Source: three-view drawing plus pictorial views. Frame: mm from the lowest corner of the part. A direction names the side the tool comes from. Give positions to 0.01 mm unless a question says otherwise; leave off trailing zeros. Loops run counter-clockwise (first coordinate to the right, second up) from the corner with the lowest first, then second, coordinate; pieces in that order, holes last.
1. Material intervals for line 1 along X through (y, z) = (29, 0.8); line 2 along X through (y, z) = (36, 14.5); line 3 along Y through (x, z) = (30, 14), sorted ascending.
2. First-contact query: P1, Ø1.5, axis at x = 15, z = 6.5, coming from the -Y side; P2, Ø6, axis at x = 31, y = 29, coming from the +Z side. Flat tips, straight axial feed; report the tip coordinate or a pass-through.
3. Section A-A, the plane y = 29. Output: boundary loops of the cut face in (x, z), then the cut area to 3 significant figures.
4. Section D-D, the plane y = 6.5. Output: boundary loops of the cut face in (x, z), then the cut area to 3 significant figures.
5. Draft query along X for the marked faces 1, 2 and 3. Return one class per face: +X half, -X half, draft (parallel to the pull), parting line (faces both ways), or undercut.
6. Section B-B, the plane x = 60.45. Output: boundary loops of the cut face in (y, z), then the cut area to 3 significant figures.
7. Access query for the marked faces 4 and 5. Directions: +Z, -Z, +X, -X, +Y, -Y. A direction counts if a zero-diameter tool reaches every point of the face in a straight line with its end or side. Return the directions, or none.
8. Section C-C, the plane z = 7.5. Output: boundary loops of the cut face in (x, y).
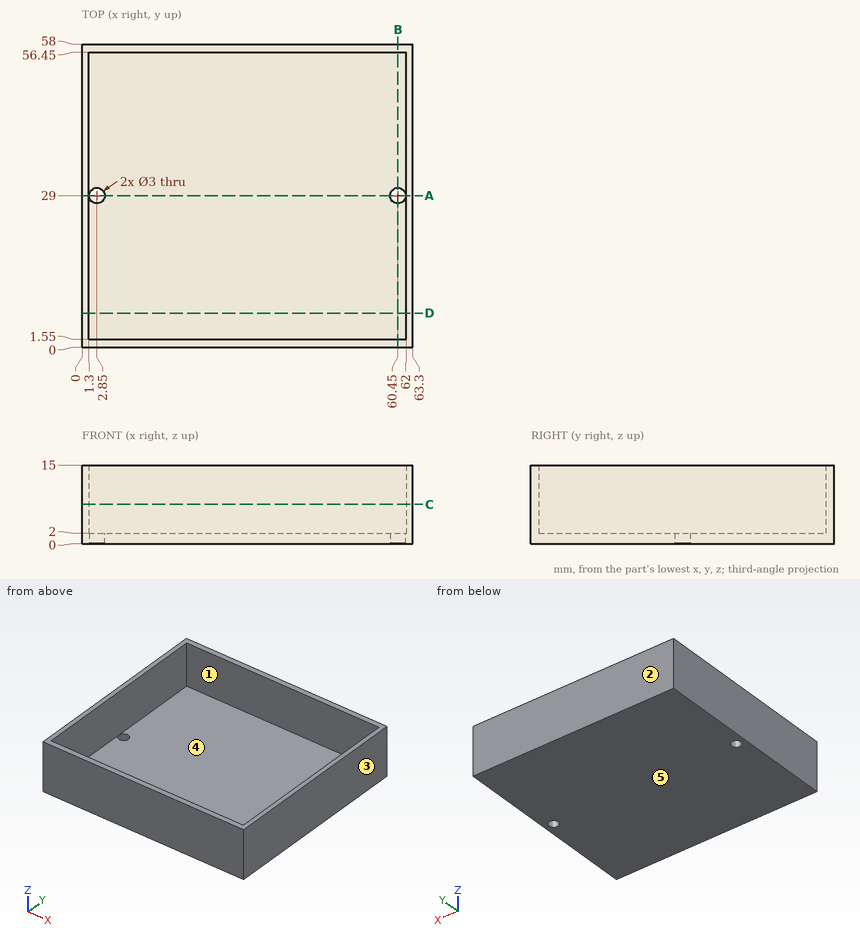
Answers below:
1. line 1: x = 0 to 1.35, 4.35 to 58.95, 61.95 to 63.3
1. line 2: x = 0 to 1.3, 62 to 63.3
1. line 3: y = 0 to 1.55, 56.45 to 58
2. P1: stops at y = 0
2. P2: stops at z = 2
3. outline: (0, 0) - (1.35, 0) - (1.35, 2) - (1.3, 2) - (1.3, 15) - (0, 15) - close; (4.35, 0) - (58.95, 0) - (58.95, 2) - (4.35, 2) - close; (61.95, 0) - (63.3, 0) - (63.3, 15) - (62, 15) - (62, 2) - (61.95, 2) - close
3. area: 148 mm2
4. outline: (0, 0) - (63.3, 0) - (63.3, 15) - (62, 15) - (62, 2) - (1.3, 2) - (1.3, 15) - (0, 15) - close
4. area: 160 mm2
5. face 1: undercut
5. face 2: draft
5. face 3: +X half
6. outline: (0, 0) - (27.5, 0) - (27.5, 2) - (1.55, 2) - (1.55, 15) - (0, 15) - close; (30.5, 0) - (58, 0) - (58, 15) - (56.45, 15) - (56.45, 2) - (30.5, 2) - close
6. area: 150 mm2
7. face 4: +Z
7. face 5: -Z, +X, -X, +Y, -Y
8. outline: (0, 0) - (63.3, 0) - (63.3, 58) - (0, 58) - close; hole (1.3, 1.55) - (62, 1.55) - (62, 56.45) - (1.3, 56.45) - close
